Geometry: see drawing. Coordinates: mm, zero at the bounding-box minimum. A direction names the side the tool comes from. Give positions to 0.01 mm unless a question says otherwise; leave off trailing zeros. Write each loop counter-clockwise with the first axis right and the second up, starting at its lowest first coordinate (ties: lowest second). Pieces come first, ordered by that corner, then holes. Notation, with made-up numbers: (84.25, -13.5) - (106.25, -13.5) arc R27 ccw to (106.25, 13.5) - close; hole circle Ø2 at (24.5, 17.5). An arc over 180 degrees is marked (long way). Use CSV: the item, a comma, the result in double quotes. Start each with the question number.
(1) Reachability of the marked faces 1, 2 and 3 from +Z, -Z, +X, -X, +Y, -Y: full face, straight path, thin tool, end or side. Return the list, or none.
(2) Section A-A on x = 5. Count the separate pieces of the cut face and the enclosed holes in it.
(3) Line query: probe 1 along Z at (x, y) = (5, 0.9) (1 decimal); probe 2 along Z at (x, y) = (5.75, 1.35); probe 3 along X at (y, z) = (0.6, 12.5). Output: solid intervals per line, ascending. Write a range as [from, to].
(4) Section C-C on x = 15. Output: boundary loops of the cut face in (y, z).
(5) Draft query along Z for the marked faces 4, 5 and 6. Return one class per face: released by +Z, released by -Z, zero draft, split by the parting line, or undercut.
(6) First-contact query: pin 1 Ø1.5 at (x, y) = (17.5, 0.5) entering from -Z; pin 2 Ø1.5 at (x, y) = (9, 1.5) entering from +Z. Flat tips, straight axial feed; report the tip coordinate or a pass-through.
(7) Section B-B on z = 18.25. Output: boundary loops of the cut face in (x, y).
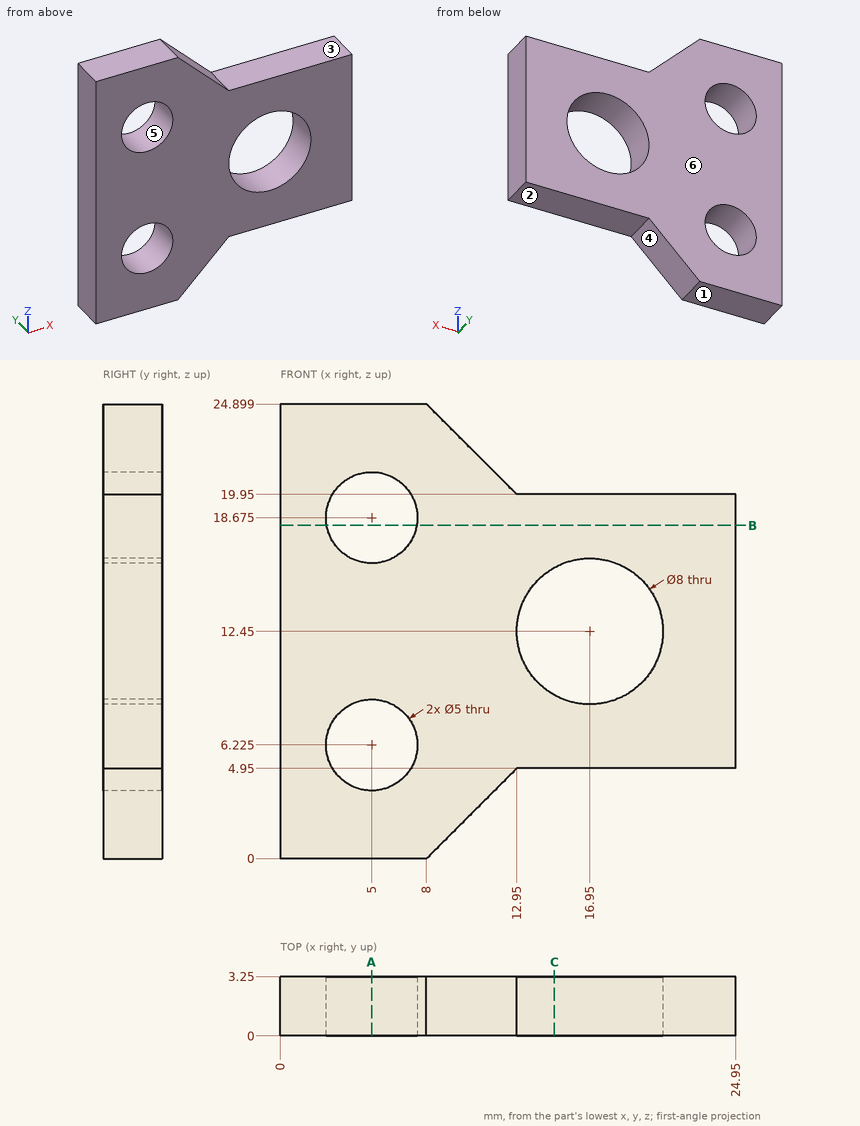
Check values:
1,face 1,"-Z, +X, -X, +Y, -Y"
1,face 2,"-Z, +X, +Y, -Y"
1,face 3,"+Z, +X, +Y, -Y"
2,separate pieces,"3"
2,enclosed holes,"0"
3,probe 1,"z = [0, 3.7], [8.7, 16.2], [21.2, 24.9]"
3,probe 2,"z = [0, 3.84], [8.61, 16.29], [21.06, 24.9]"
3,probe 3,"x = [0, 12.95], [20.95, 24.95]"
4,outline,"(0, 4.95) - (3.25, 4.95) - (3.25, 8.96) - (0, 8.96) - close; (0, 15.94) - (3.25, 15.94) - (3.25, 19.95) - (0, 19.95) - close"
5,face 4,"released by -Z"
5,face 5,"undercut"
5,face 6,"zero draft"
6,pin 1,"stops at z = 4.95"
6,pin 2,"stops at z = 24.65"
7,outline,"(0, 0) - (2.54, 0) - (2.54, 3.25) - (0, 3.25) - close; (7.46, 0) - (24.95, 0) - (24.95, 3.25) - (7.46, 3.25) - close"
